```python
from build123d import *

# Parameters (mm, degrees)
EXTRUDE_THIN1_DEPTH = 762
FILLET1_R           = 1.651


with BuildPart() as part:
    # Sketch1 → Extrude-Thin1 (new body)
    with BuildSketch(Plane.XY):
        with BuildLine():
            Line((0, 0), (0, 8.73125))
            Line((0, 8.73125), (-5.55625, 8.73125))
            Line((-5.55625, 8.73125), (-5.55625, 15.08125))
            ThreePointArc((-5.55625, 15.08125), (-16.235064, 19.837192), (-19.84375, 30.95625))
            Line((-19.84375, 30.95625), (-38.89375, 30.95625))
            Line((-38.89375, 30.95625), (-38.89375, 56.35625))
            ThreePointArc((-38.89375, 56.35625), (-39.341606, 57.151515), (-40.253834, 57.180844))
            ThreePointArc((-40.253834, 57.180844), (-41.798306, 57.35168), (-42.225966, 58.845562))
            ThreePointArc((-42.225966, 58.845562), (-42.493091, 62.371576), (-45.152095, 64.702632))
            ThreePointArc((-45.152095, 64.702632), (-47.13073, 66.482003), (-47.230922, 69.14116))
            ThreePointArc((-47.230922, 69.14116), (-47.420593, 70.70524), (-48.815625, 71.4375))
            Line((-48.815625, 71.4375), (-50.8, 71.4375))
            Line((-50.8, 71.4375), (-50.8, 79.375))
            Line((-50.8, 79.375), (-32.823706, 79.375))
            Line((-32.823706, 79.375), (-32.823706, 77.724))
            Line((-32.823706, 77.724), (-49.149, 77.724))
            Line((-49.149, 77.724), (-49.149, 73.0885))
            Line((-49.149, 73.0885), (-48.815625, 73.0885))
            ThreePointArc((-48.815625, 73.0885), (-46.061751, 71.642976), (-45.68733, 68.555392))
            ThreePointArc((-45.68733, 68.555392), (-45.635593, 67.182265), (-44.613871, 66.263439))
            ThreePointArc((-44.613871, 66.263439), (-41.137974, 63.341171), (-40.514728, 58.843051))
            ThreePointArc((-40.514728, 58.843051), (-38.261995, 58.411123), (-37.24275, 56.35625))
            Line((-37.24275, 56.35625), (-37.24275, 32.60725))
            Line((-37.24275, 32.60725), (-17.87345, 32.60725))
            ThreePointArc((-17.87345, 32.60725), (-15.074359, 21.016098), (-3.90525, 16.839887))
            Line((-3.90525, 16.839887), (-3.90525, 10.38225))
            Line((-3.90525, 10.38225), (1.651, 10.38225))
            Line((1.651, 10.38225), (1.651, 0))
            Line((1.651, 0), (0, 0))
        make_face()
    extrude(amount=-EXTRUDE_THIN1_DEPTH)

    # Fillet1
    fillet1_edges = [part.edges().sort_by_distance(p)[0] for p in [
        (-17.87345, 32.60725, -381),
        (-3.90525, 16.839887, -381),
        (1.651, 10.38225, -381),
        (-5.55625, 8.73125, -381),
        (-38.89375, 30.95625, -381),
        (-50.8, 71.4375, -381),
        (-50.8, 79.375, -381),
    ]]
    fillet(fillet1_edges, radius=FILLET1_R)


solid = part.part
```
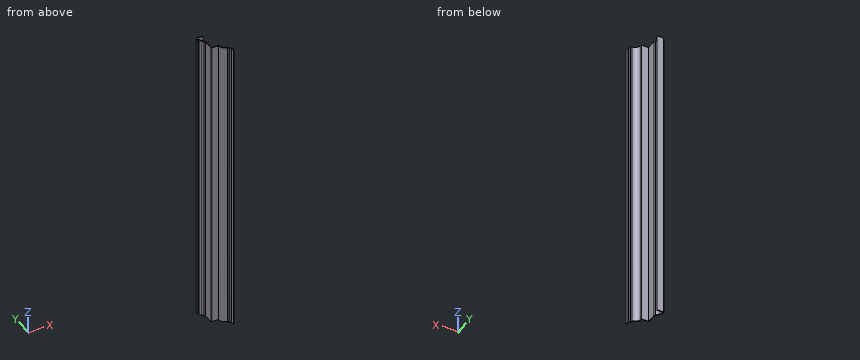
Verification items for the finished model (mm, model axes). Coordinates: 2 decimals unless noted, no trailing zeros. Order: outer loops, then holes, each group sorted by start corner. A loop starts at its lowest first (then second) coordinate and runs counter-clockwise, first axis right, second up. Notation, with made-up numbers: (89.5, 29) -> (118.5, 29) arc R30 cw to (118.5, 66) -> close; hole circle Ø5 at (22.25, 8). An arc over 180 degrees is marked (long way). Answer as CSV lines item,"result". Start each with the question number.
1) Material ranges on L1, parallel to X at y = 36.5, z = -416; L2, parallel to Y at x = -38.5, z = -239 (3 decimals); L3, parallel to Y at x = -45, z = -121 (3 decimals), recorded low to high. Write a range as [from, to].
2) Gauge pin test, flat ends, axial feed: pin 1 Ø2.5 at (y, z) = (75.5, -276) entering from +X; pin 2 Ø3 at (y, z) = (25, -176) entering from +X; pin 3 Ø1.4 at (y, z) = (11.5, -434.5) entering from -X; pin 4 Ø8 at (x, y) = (-31, 44.5) entering from -Z. Record the tip position at first contact, or that the pin passes through.
3) Cross-section at A-A, the plane y = 46.5. Record the boundary of the cut face in (x, z), then the cut area to 3 significant figures.
Conclusion:
1,L1,"x = [-38.89, -37.24]"
1,L2,"y = [31.537, 58.572], [77.724, 79.375]"
1,L3,"y = [64.647, 66.452], [77.724, 79.375]"
2,pin 1,"stops at x = -49.15"
2,pin 2,"stops at x = -16.8"
2,pin 3,"stops at x = -5.56"
2,pin 4,"passes through"
3,outline,"(-38.89, -762) -> (-37.24, -762) -> (-37.24, 0) -> (-38.89, 0) -> close"
3,area,"1,260 mm²"
